Here's how the part is built. I have some questions about the finished solid (model axes, mm). A direction names the side the tool comes from. Coordinates: 2 decimals unless noted, no trailing zeros. Write each loop counter-clockwise with the first axis right and the second up, starting at its lowest first coordinate (ties: lowest second). Pieces come first, ordered by that corner, then holes. Notation, with made-up numbers: (69.25, -33.5) - (76.25, -33.5) arc R24 cw to (76.25, -20.5) - close; hole circle Ø4 at (82, 6). An arc over 180 degrees is marked (long way). Answer in a Markdown table with one row per item. Add a question column.
Item 1: Imagine slicing it at D-D (z = -3). Please give me the cut outline in (x, y), plus the area to 3 significant figures.
Item 2: We'd pull the mould along X, two halves only. Please class faces 3 (the face through (0.27, -1.22, 32.18)), 4 (the face through (0, -8, 0)), 5 (the face through (7.154, -2.253, -27.885)): +X half, -X half, draft (parallel to the pull), parting line (faces both ways), or undercut.
Item 3: Imagine slicing it at C-C (y = -4.75). Please give me the cut outline in (x, z).
Item 4: Imagine slicing it at A-A (x = -4.25). Please give me the cut outline in (y, z).
Item 5: I'm going to push flat-ended pins straight in: pin 1 (1.5 mm diameter, centred on y = 6, z = 8.5, fed in from +X); pin 2 (1 mm diameter, centred on x = -4, z = -33.5, fed in from -Y); pin 3 (8 mm diameter, centred on y = -6.5, z = -10.5, fed in from +X). Where does each tip first touch, or does it pass through?
Item 6: Imagine slicing it at B-B (z = 33). Please give me the cut outline in (x, y).
Item 7: If I drill on probe 1 along Z at (x, y) = (-2, 0); probe 2 along X at (y, z) = (0, 34); probe 3 along Y at (x, z) = (4.25, -27.5), over which ranges is the centre line in solid material (lowest first)? Write a range as from..to.
Item 8: Which directions (+Z, -Z, +X, -X, +Y, -Y) give clear straight access to the entire face, cutting with the end or side of a thin tool? Please do faces 1 (the face through (-7.493, 0.33, 24.79)), 2 (the face through (11.923, 3.755, 4.93)).
from build123d import *

# Parameters (mm, degrees)
SKETCH1_R                       = 12.5
F_25MM_DIA_DEPTH                = 10
F_15MM_START                    = -10
SKETCH2_R                       = 7.5
F_15MM_DIA_BEARING_END_DEPTH    = 40
F_15MM_START_2                  = 55
SKETCH3_R                       = 7.5
F_15MM_DIA_GEAR_END_DEPTH       = 55
M3X0_5_TAPPED_HOLE1_D           = 2.5
M3X0_5_TAPPED_HOLE1_DEPTH       = 15
M3X0_5_TAPPED_HOLE1_CSINK_D     = 4
M3X0_5_TAPPED_HOLE1_CSINK_ANGLE = 120
M3X0_5_TAPPED_HOLE1_TIP         = 0.751075774
SKETCH7_R                       = 2
CUT_EXTRUDE1_DEPTH              = 60.843546018


with BuildPart() as part:
    # Sketch1 → 25mm dia (new body)
    with BuildSketch(Plane.XY):
        Circle(SKETCH1_R)
    extrude(amount=F_25MM_DIA_DEPTH)

    # Sketch2 → 15mm dia bearing end (add)
    with BuildSketch(Plane.XY.offset(10).offset(F_15MM_START)):
        Circle(SKETCH2_R)
    extrude(amount=F_15MM_DIA_BEARING_END_DEPTH)

    # Sketch3 → 15mm dia gear end (add)
    with BuildSketch(Plane(origin=(0, 0, 0), x_dir=(-1, 0, 0), z_dir=(0, 0, -1)).offset(F_15MM_START_2)):
        with Locations(Location((0, 0, 0), (0, 0, 180))):
            Circle(SKETCH3_R)
    extrude(amount=-F_15MM_DIA_GEAR_END_DEPTH)

    # M3x0.5 Tapped Hole1
    with Locations(Plane.XY.offset(40)):
        with Locations((0, 0)):
            CounterSinkHole(M3X0_5_TAPPED_HOLE1_D / 2, M3X0_5_TAPPED_HOLE1_CSINK_D / 2, depth=M3X0_5_TAPPED_HOLE1_DEPTH, counter_sink_angle=M3X0_5_TAPPED_HOLE1_CSINK_ANGLE)
            with Locations((0, 0, -(M3X0_5_TAPPED_HOLE1_DEPTH + M3X0_5_TAPPED_HOLE1_TIP / 2))):  # 118° drill point
                Cone(0, M3X0_5_TAPPED_HOLE1_D / 2, M3X0_5_TAPPED_HOLE1_TIP, mode=Mode.SUBTRACT)

    # Sketch7 → Cut-Extrude1 (cut, through all)
    with BuildSketch(Plane(origin=(7.5, 0, 0), x_dir=(0, 0, -1), z_dir=(1, 0, 0))):
        with Locations((27.5, 0)):
            Circle(SKETCH7_R)
    extrude(amount=-CUT_EXTRUDE1_DEPTH, mode=Mode.SUBTRACT)


solid = part.part
Here are the results:
| question | item | result |
|---|---|---|
| 1 | outline | circle Ø15 at (0, 0) |
| 1 | area | 177 mm2 |
| 2 | face 3 | undercut |
| 2 | face 4 | draft |
| 2 | face 5 | parting line |
| 3 | outline | (-11.56, 0) - (-5.8, 0) - (-5.8, -55) - (5.8, -55) - (5.8, 0) - (11.56, 0) - (11.56, 10) - (5.8, 10) - (5.8, 40) - (-5.8, 40) - (-5.8, 10) - (-11.56, 10) - close |
| 4 | outline | (-11.76, 0) - (-6.18, 0) - (-6.18, -55) - (6.18, -55) - (6.18, 0) - (11.76, 0) - (11.76, 10) - (6.18, 10) - (6.18, 40) - (-6.18, 40) - (-6.18, 10) - (-11.76, 10) - close; hole circle Ø4 at (0, -27.5) |
| 5 | pin 1 | stops at x = 11.34 |
| 5 | pin 2 | stops at y = -6.63 |
| 5 | pin 3 | stops at x = 7.07 |
| 6 | outline | circle Ø15 at (0, 0); hole circle Ø2.5 at (0, 0) |
| 7 | probe 1 | z = -55..-29.5, -25.5..40 |
| 7 | probe 2 | x = -7.5..-1.25, 1.25..7.5 |
| 7 | probe 3 | y = -6.18..-2, 2..6.18 |
| 8 | face 1 | +Z |
| 8 | face 2 | +Z, -Z |
